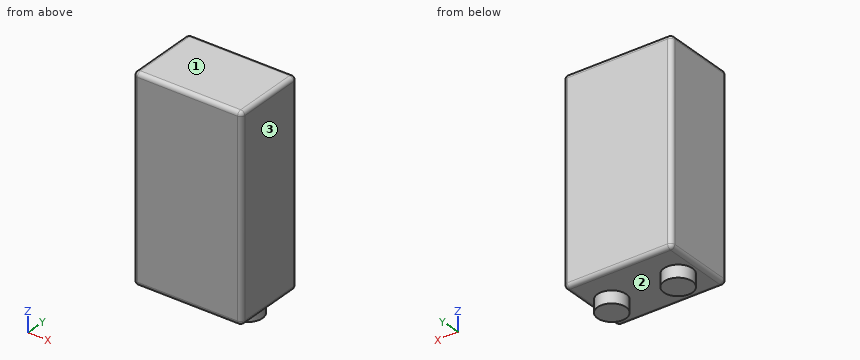
```python
from build123d import *

# Parameters (mm, degrees)
ESQUISSE1_W        = 26.5
ESQUISSE1_H        = 49
BOSS_EXTRU_1_DEPTH = 18
CONG_1_R           = 1
ESQUISSE2_R        = 3.5
BOSS_EXTRU_2_DEPTH = 3


with BuildPart() as part:
    # Esquisse1 → Boss.-Extru.1 (new body)
    with BuildSketch(Plane(origin=(0, 0, 0), x_dir=(1, 0, 0), z_dir=(0, 1, 0))):
        Rectangle(ESQUISSE1_W, ESQUISSE1_H)
    extrude(amount=BOSS_EXTRU_1_DEPTH)

    # Congé1
    cong_1_edges = [part.edges().sort_by_distance(p)[0] for p in [
        (-13.25, 18, 0),
        (0, 18, 24.5),
        (13.25, 18, 0),
        (0, 0, 24.5),
        (-13.25, 0, 0),
        (0, 0, -24.5),
        (13.25, 0, 0),
        (13.25, 9, 24.5),
        (-13.25, 9, 24.5),
        (-13.25, 9, -24.5),
        (13.25, 9, -24.5),
        (0, 18, -24.5),
    ]]
    fillet(cong_1_edges, radius=CONG_1_R)

    # Esquisse2 → Boss.-Extru.2 (add)
    with BuildSketch(Plane(origin=(0, 0, -24.5), x_dir=(-1, 0, 0), z_dir=(0, 0, -1))):
        with Locations(Location((-8.113267723, 9, 0), (0, 0, 180))):
            Circle(ESQUISSE2_R)
    boss_extru_2 = extrude(amount=BOSS_EXTRU_2_DEPTH)

    # Symétrie1: Boss.-Extru.2 across plane
    add(boss_extru_2.mirror(Plane(origin=(0, 0, 0), x_dir=(0, 0, 1), z_dir=(1, 0, 0))))


solid = part.part
```
Build history of the part. All positions in model axes, mm. Face numbers are marked on the shaded views. Give positions to 0.01 mm unless a question says otherwise; leave off trailing zeros. Loops run counter-clockwise (first coordinate to the right, second up) from the corner with the lowest first, then second, coordinate; pieces in that order, holes last.
1) Band-saw the part on B-B on y = 15.75. List the corners of the cut face in (x, z), then the cut area to 3 significant figures.
Values follow:
outline: (-13.25, -23.5) arc R1 ccw to (-12.25, -24.5) - (12.25, -24.5) arc R1 ccw to (13.25, -23.5) - (13.25, 23.5) arc R1 ccw to (12.25, 24.5) - (-12.25, 24.5) arc R1 ccw to (-13.25, 23.5) - close
area: 1,300 mm2
2) Probe line 1 along Z through (x, y) = (-0.5, 8.5). List the from-to ranges inside material, lowest first.
Values follow:
line 1: z = -24.5 to 24.5
3) Drop a flat-ended pin along its axis: P1, Ø5, axis at x = 6.5, y = 2.5, coming from the -Z side. Give the stop position or say it passes through.
Values follow:
P1: stops at z = -24.5
4) Band-saw the part on C-C on x = 0. List the corners of the cut face in (y, z).
Values follow:
outline: (0, -23.5) arc R1 ccw to (1, -24.5) - (17, -24.5) arc R1 ccw to (18, -23.5) - (18, 23.5) arc R1 ccw to (17, 24.5) - (1, 24.5) arc R1 ccw to (0, 23.5) - close
5) Band-saw the part on A-A on x = 6. List the corners of the cut face in (y, z), then the cut area to 3 significant figures.
Values follow:
outline: (0, -23.5) arc R1 ccw to (1, -24.5) - (6.21, -24.5) - (6.21, -27.5) - (11.79, -27.5) - (11.79, -24.5) - (17, -24.5) arc R1 ccw to (18, -23.5) - (18, 23.5) arc R1 ccw to (17, 24.5) - (1, 24.5) arc R1 ccw to (0, 23.5) - close
area: 898 mm2
6) Two-plate mould, pull along X, no slides. Class the marked faces 1, 2 and 3: released by +X, released by -X, zero draft, split by the parting line, or undercut.
Values follow:
face 1: zero draft
face 2: undercut
face 3: released by +X
7) Band-saw the part on D-D on y = 6.5. List the corners of the cut face in (x, z).
Values follow:
outline: (-13.25, -23.5) arc R1 ccw to (-12.25, -24.5) - (-10.56, -24.5) - (-10.56, -27.5) - (-5.66, -27.5) - (-5.66, -24.5) - (5.66, -24.5) - (5.66, -27.5) - (10.56, -27.5) - (10.56, -24.5) - (12.25, -24.5) arc R1 ccw to (13.25, -23.5) - (13.25, 23.5) arc R1 ccw to (12.25, 24.5) - (-12.25, 24.5) arc R1 ccw to (-13.25, 23.5) - close
